Geometry check sheet. Reference: the model listing, model coordinates, mm. A direction names the side the tool comes from. Round coordinates to 2 decimals unless told otherwise and drop trailing zeros. Order: outer loops, then holes, each group sorted by start corner. A loop starts at its lowest first (then second) coordinate and runs counter-clockwise, first axis right, second up.
(1) Cross-section at B-B on z = 2. Enter the section's corners in (x, y).
(2) Thickness scan on L1, parallel to Y at x = -1.1, z = -18.6; L2, parallel to Z at x = -7, y = 12; L3, parallel to Z at x = -2, y = 14.5. Record the ranges inside material, lowest first.
(3) Set-up check for faces 4 (the face through (-1.48, 13.08, -9.42)), 5 (the face through (-9.458, 12.13, -7.653)): record each of +Z, -Z, +X, -X, +Y, -Y from which the full face is reachable in a straight line by a thin tool's end or side.
(4) Cross-section at A-A on x = -2. Enter the section's corners in (y, z).
(5) Cross-section at D-D on z = -26.6. Enter the section's corners in (x, y).
(6) Cross-section at C-C on y = 20. Enter the section's corners in (x, z).
(7) Gauge pin test, flat ends, axial feed: P1, Ø1, axis at x = -11.5, z = -22.5, coming from the -Y side; P2, Ø4.5, axis at y = 12, z = -26.6, coming from the -X side; P3, Ø3, axis at y = 17, z = -16, coming from the +X side; P4, Ø1, axis at y = 9.5, z = -2, coming from the -X side. Record the tip position at first contact, or that the pin passes through.
(8) Draft check along X on faces 1 (the face through (-8, 0, -9)), 2 (the face through (-19.1, 12.2, 2)), 3 (the face through (-3, 2.7, -19.9)). Enter one of: pulls with the +X half, pulls with the -X half, needs draft (parallel to the pull), parting line crosses it, or undercut.
Autodesk Inventor part; units mm, degrees
ref_plane "Work Plane1" through (-3, 0, 4) normal (1, 0, 0) x (0, 0, -1)
ref_plane "YZ Plane" through (0, 0, 0) normal (1, 0, 0) x (0, 1, 0)
ref_plane "XZ Plane" through (0, 0, 0) normal (0, 1, 0) x (-1, 0, 0)
sketch "Sketch1" plane through (0, 0, 0) normal (0, 1, 0) x (-1, 0, 0)
  line L0 (0, 0) -> (0, -30.6)
  line L1 (0, -30.6) -> (5, -30.6)
  line L2 (0, 0) -> (19.774, 0)
  line L3 (19.774, 0) -> (5, -30.6)
  line L4 (19.774, 0) -> (19.774, 4)
  line L5 (0, 0) -> (0, 9.5471)
  line L6 (19.774, 4) -> (-4.8744, 4)
  point P0 (0, 4)
  dimension "d0" = 30.6
  dimension "d1" = 5
  dimension "d2" = 19.774
  dimension "d3" = 4
extrude "Extrusion1" add sketch "Sketch1" along normal blind 24
sketch "Sketch2" plane through (0, 0, 4) normal (1, 0, 0) x (0, 0, -1)
  line L0 (34.6, 0) -> (34.6, 24)
  line L1 (34.6, 12) -> (30.6, 12)
  line L2 (30.6, 12) -> (14.6, 12)
  line L3 (22.6, 12) -> (22.6, 20)
  line L4 (22.6, 12) -> (22.6, 4)
  circle A0 centre (22.6, 20) radius 1.6
  circle A1 centre (14.6, 12) radius 1.6
  circle A2 centre (22.6, 4) radius 1.6
  circle A3 centre (30.6, 12) radius 1.6
  point P0 (4, 0)
  dimension "d6" = 4
  dimension "d7" = 16
  dimension "d8" = 8
  dimension "d9" = 8
  dimension "d10" = 3.2
  dimension "d11" = 3.2
  dimension "d12" = 3.2
  dimension "d13" = 3.2
extrude "Extrusion2" cut sketch "Sketch2" against normal blind 24
ref_plane "Work Plane1" through (-3, 0, 4) normal (1, 0, 0) x (0, 0, -1)
sketch "Sketch3" plane through (-3, 0, 4) normal (1, 0, 0) x (0, 0, -1)
  circle A0 centre (22.6, 20) radius 1.6
  circle A1 centre (22.6, 20) radius 2.95
  circle A2 centre (14.6, 12) radius 1.6
  circle A3 centre (14.6, 12) radius 2.95
  circle A4 centre (22.6, 4) radius 1.6
  circle A5 centre (22.6, 4) radius 2.95
  circle A6 centre (30.6, 12) radius 1.6
  circle A7 centre (30.6, 12) radius 2.95
  point P0 (4, 0)
  dimension "d17" = 5.9
  dimension "d18" = 5.9
  dimension "d19" = 5.9
  dimension "d20" = 5.9
extrude "Extrusion3" cut sketch "Sketch3" against normal blind 24 contours A0 | A1 | A2 | A3 | A4 | A5 | A6 | A7
sketch "Sketch4" plane through (0, 24, 0) normal (0, 1, 0) x (1, 0, 0)
  line L0 (0, -4) -> (0, 30.6)
  line L1 (0, -4) -> (-2, -4)
  line L2 (-2, -4) -> (-2, -2)
  line L3 (-2, -2) -> (0, -2)
  line L4 (0, -2) -> (0, -4)
  circle A0 centre (-2, -2) radius 1.1
  line L5 (-2, -2) -> (-18, -2)
  circle A1 centre (-18, -2) radius 1.1
  point P0 (0, 0)
  dimension "d23" = 2
  dimension "d24" = 2
  dimension "d25" = 2.2
  dimension "d26" = 16
  dimension "d27" = 2.2
extrude "Extrusion4" cut sketch "Sketch4" against normal blind 24 contours A1 | A0 L2 L3 | L3 L5 A0 | A0 L5 L2
properties part number "Finger_right_v5"
Found:
1. outline: (-19.77, 0) - (-19.1, 0) - (-19.1, 24) - (-19.77, 24) - close; (-16.9, 0) - (-3.1, 0) - (-3.1, 24) - (-16.9, 24) - close; (-0.9, 0) - (0, 0) - (0, 24) - (-0.9, 24) - close
2. L1: y = 0 to 2.4, 5.6 to 18.4, 21.6 to 24
2. L2: z = -23.65 to -13.55, -7.65 to 4
2. L3: z = -30.6 to 0.9, 3.1 to 4
3. face 4: +X, -X
3. face 5: -X
4. outline: (0, -30.6) - (24, -30.6) - (24, 0.9) - (0, 0.9) - close; (0, 3.1) - (24, 3.1) - (24, 4) - (0, 4) - close; hole circle Ø3.2 at (4, -18.6); hole circle Ø3.2 at (12, -26.6); hole circle Ø3.2 at (12, -10.6); hole circle Ø3.2 at (20, -18.6)
5. outline: (-6.93, 0) - (0, 0) - (0, 10.4) - (-3, 10.4) - (-3, 9.05) - (-6.93, 9.05) - close; (-6.93, 14.95) - (-3, 14.95) - (-3, 13.6) - (0, 13.6) - (0, 24) - (-6.93, 24) - close
6. outline: (-19.77, 0) - (-12.22, -15.65) - (-3, -15.65) - (-3, -17) - (0, -17) - (0, 4) - (-19.77, 4) - close; (-9.37, -21.55) - (-5, -30.6) - (0, -30.6) - (0, -20.2) - (-3, -20.2) - (-3, -21.55) - close; hole circle Ø2.2 at (-18, 2); hole circle Ø2.2 at (-2, 2)
7. P1: passes through
7. P2: stops at x = -3
7. P3: stops at x = 0
7. P4: stops at x = -19.05
8. face 1: needs draft
8. face 2: undercut
8. face 3: pulls with the -X half
